Design review of the part shown in the three views and the two pictorial views. Dimensions are in mm from the part's minimum x, y and z. Give positions to 0.01 mm unless a question says otherwise; leave off trailing zeros. Loops run counter-clockwise (first coordinate to the right, second up) from the corner with the lowest first, then second, coordinate; pieces in that order, holes last. Notation, with made-up numbers: (-39.75, 71) - (-24.75, 71) arc R17 ccw to (-24.75, 75) - close; hole circle Ø7 at (-33, 74). An arc over 180 degrees is marked (long way). Answer in a Markdown table with one row per item.
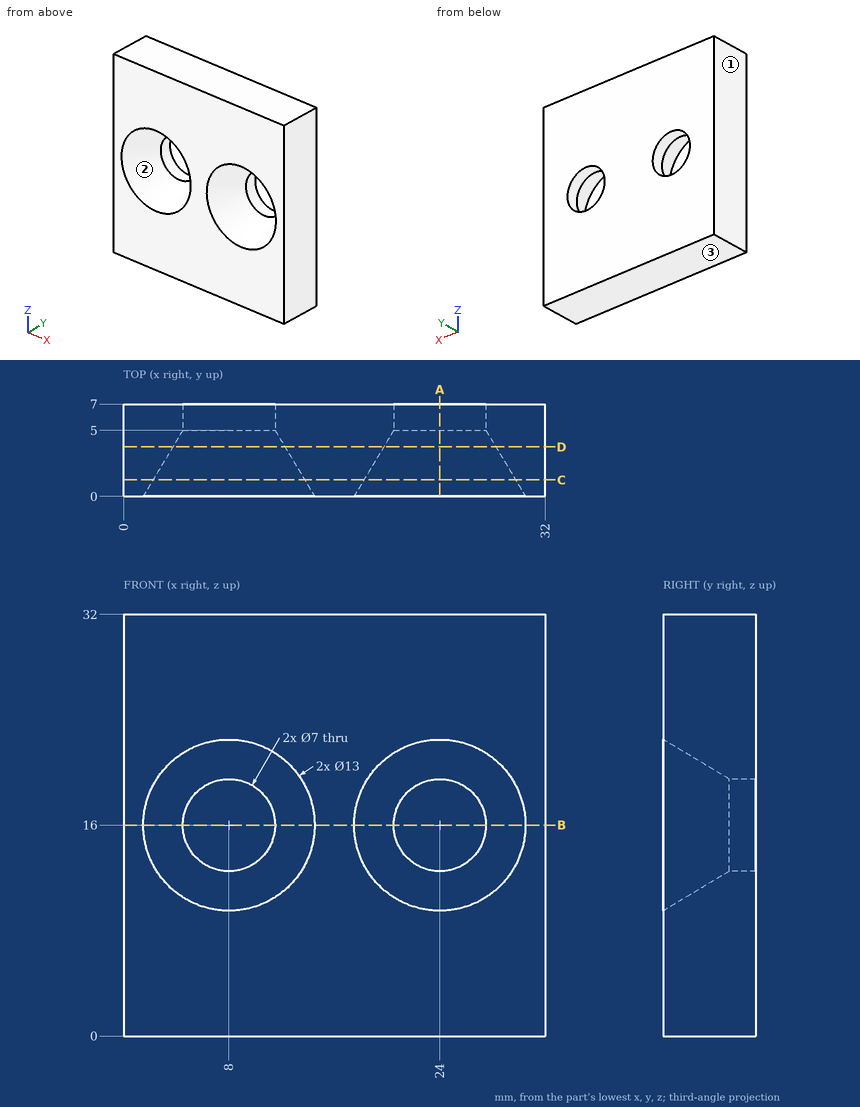
1. We need section A-A, the plane x = 24. Give the boundary of the cut face in (y, z).
Values:
| item | result |
|---|---|
| outline | (0, 0) - (7, 0) - (7, 12.5) - (5, 12.5) - (0, 9.5) - close; (0, 22.5) - (5, 19.5) - (7, 19.5) - (7, 32) - (0, 32) - close |
2. We need section D-D, the plane y = 3.75. Give the boundary of the cut face in (x, z).
Values:
| item | result |
|---|---|
| outline | (0, 0) - (32, 0) - (32, 32) - (0, 32) - close; hole circle Ø8.5 at (8, 16); hole circle Ø8.5 at (24, 16) |
3. We need section C-C, the plane y = 1.25. Give the boundary of the cut face in (x, z).
Values:
| item | result |
|---|---|
| outline | (0, 0) - (32, 0) - (32, 32) - (0, 32) - close; hole circle Ø11.5 at (8, 16); hole circle Ø11.5 at (24, 16) |
4. Wall thickness on line 1 (X direction, y = 5.7, z = 16); line 2 (Z direction, x = 8, y = 6.25); line 3 (X direction, y = 1, z = 16.5): over which ranges is each line inside the solid? List them lowest first. Write a range as [from, to].
Values:
| item | result |
|---|---|
| line 1 | x = [0, 4.5], [11.5, 20.5], [27.5, 32] |
| line 2 | z = [0, 12.5], [19.5, 32] |
| line 3 | x = [0, 2.12], [13.88, 18.12], [29.88, 32] |
5. We need section B-B, the plane z = 16. Give the boundary of the cut face in (x, y), and give its area (3 significant figures).
Values:
| item | result |
|---|---|
| outline | (0, 0) - (1.5, 0) - (4.5, 5) - (4.5, 7) - (0, 7) - close; (11.5, 5) - (14.5, 0) - (17.5, 0) - (20.5, 5) - (20.5, 7) - (11.5, 7) - close; (27.5, 5) - (30.5, 0) - (32, 0) - (32, 7) - (27.5, 7) - close |
| area | 96.0 mm^2 |
6. Mouldability with a two-part tool opening along X and no side actions: class the marked faces 1, 2 and 3 as released by +X, released by -X, zero draft, split by the parting line, or undercut.
Values:
| item | result |
|---|---|
| face 1 | released by -X |
| face 2 | undercut |
| face 3 | zero draft |
